The model under review builds one solid part; all positions refer to its coordinate system, in mm. A direction names the side the tool comes from. Round coordinates to 2 decimals unless told otherwise and drop trailing zeros. Write each loop counter-clockwise with the first axis right and the second up, starting at its lowest first coordinate (ties: lowest second). Pieces come first, ordered by that corner, then holes.
Item 1: Add section A-A (x = -20). Give the boundary of the cut face in (y, z).
Item 2: Add section B-B (z = 2.75). Give the boundary of the cut face in (x, y), plus the area to 3 significant figures.
Item 3: Add section D-D (x = -12). Give the boundary of the cut face in (y, z), plus the area to 3 significant figures.
Item 4: Add section C-C (y = 46). Give the boundary of the cut face in (x, z), plus the area to 3 significant figures.
Item 5: To check wall thickness, follow L1, parallel to Y at x = 20, z = 2.35; L2, parallel to Y at x = -19, z = 7; L3, parallel to X at y = -47, z = 3. State the ranges of each line that lie inside material, in increasing order.
Item 6: Machinability: for faces 1 (the face through (0, 46, 4)), 2 (the face through (0, -28, 6)), 3 (the face through (10, -46, 2)), 4 (the face through (18, -46, 4)), which of the approach directions +Z, -Z, +X, -X, +Y, -Y give a long, thin tool a straight path to every point of the face, cutting with its end or side? Answer none if there is none.
Item 7: Clearance check with flat-ended pins moving along their axes: pin 1 Ø5 at (x, y) = (20, -46) entering from +Z; pin 2 Ø1 at (x, y) = (17.5, -35.5) entering from -Z; pin 3 Ø1.5 at (x, z) = (-12.5, 6) entering from +Y; pin 4 Ø2.5 at (x, y) = (20, 46) entering from +Z. State where each tip first meets the part, or that it passes through.
```python
from build123d import *

# Parameters (mm, degrees)
SALIENTE_EXTRUIR1_DEPTH = 4
CROQUIS2_W              = 60
CROQUIS2_H              = 8
SALIENTE_EXTRUIR2_DEPTH = 5
CROQUIS3_R              = 1.55
CROQUIS3_R_2            = 1.5
CORTAR_EXTRUIR1_DEPTH   = 64.725975865


with BuildPart() as part:
    # Croquis1 → Saliente-Extruir1 (new body)
    with BuildSketch(Plane.XY):
        Polygon((10, -36), (10, -56), (30, -56), (30, 56), (-30, 56), (-30, -56), (-10, -56), (-10, -36), align=None)
    extrude(amount=SALIENTE_EXTRUIR1_DEPTH)

    # Croquis2 → Saliente-Extruir2 (add)
    with BuildSketch(Plane.XY.offset(4)):
        with Locations((0, 32)):
            Rectangle(CROQUIS2_W, CROQUIS2_H)
        with Locations((0, -32)):
            Rectangle(CROQUIS2_W, CROQUIS2_H)
    extrude(amount=SALIENTE_EXTRUIR2_DEPTH)

    # Croquis3 → Cortar-Extruir1 (cut, through all)
    with BuildSketch(Plane.XY.offset(4)):
        with Locations((-20, -46)):
            Circle(CROQUIS3_R)
        with Locations((20, -46)):
            Circle(CROQUIS3_R)
        with Locations((-20, 46)):
            Circle(CROQUIS3_R_2)
        with Locations((20, 46)):
            Circle(CROQUIS3_R_2)
    extrude(amount=-CORTAR_EXTRUIR1_DEPTH, mode=Mode.SUBTRACT)


solid = part.part
```
Numbers:
1. outline: (-56, 0) - (-47.55, 0) - (-47.55, 4) - (-56, 4) - close; (-44.45, 0) - (44.5, 0) - (44.5, 4) - (36, 4) - (36, 9) - (28, 9) - (28, 4) - (-28, 4) - (-28, 9) - (-36, 9) - (-36, 4) - (-44.45, 4) - close; (47.5, 0) - (56, 0) - (56, 4) - (47.5, 4) - close
2. outline: (-30, -56) - (-10, -56) - (-10, -36) - (10, -36) - (10, -56) - (30, -56) - (30, 56) - (-30, 56) - close; hole circle Ø3.1 at (-20, -46); hole circle Ø3 at (-20, 46); hole circle Ø3.1 at (20, -46); hole circle Ø3 at (20, 46)
2. area: 6,290 mm2
3. outline: (-56, 0) - (56, 0) - (56, 4) - (36, 4) - (36, 9) - (28, 9) - (28, 4) - (-28, 4) - (-28, 9) - (-36, 9) - (-36, 4) - (-56, 4) - close
3. area: 528 mm2
4. outline: (-30, 0) - (-21.5, 0) - (-21.5, 4) - (-30, 4) - close; (-18.5, 0) - (18.5, 0) - (18.5, 4) - (-18.5, 4) - close; (21.5, 0) - (30, 0) - (30, 4) - (21.5, 4) - close
4. area: 216 mm2
5. L1: y = -56 to -47.55, -44.45 to 44.5, 47.5 to 56
5. L2: y = -36 to -28, 28 to 36
5. L3: x = -30 to -21.18, -18.82 to -10, 10 to 18.82, 21.18 to 30
6. face 1: +Z, +X, -X, +Y
6. face 2: +Z, +X, -X
6. face 3: +Z, -Z, -Y
6. face 4: +Z, +X, -X, -Y
7. pin 1: stops at z = 4
7. pin 2: stops at z = 0
7. pin 3: stops at y = 36
7. pin 4: passes through
